Autodesk Inventor part; units mm, degrees
ref_plane "YZ Plane" through (0, 0, 0) normal (1, 0, 0) x (0, 1, 0)
ref_plane "XZ Plane" through (0, 0, 0) normal (0, 1, 0) x (-1, 0, 0)
ref_plane "XY Plane" through (0, 0, 0) normal (0, 0, 1) x (1, 0, 0)
sketch "Sketch1" plane through (0, 0, 0) normal (0, 0, 1) x (1, 0, 0)
  line L0 (0, 6.35) -> (0, 53.34)
  line L1 (0, 53.34) -> (-19.05, 53.34)
  line L2 (-19.05, 53.34) -> (-19.05, 55.245)
  line L3 (-12.7, 48.895) -> (-6.35, 48.895)
  line L4 (-6.35, 48.895) -> (-6.35, 13.335)
  line L5 (-6.35, 13.335) -> (-19.05, 13.335)
  line L6 (-19.05, 13.335) -> (-19.05, 12.7)
  line L7 (-12.7, 8.89) -> (-6.35, 8.89)
  line L8 (-6.35, 8.89) -> (-6.35, 0)
  line L9 (-6.35, 0) -> (0, 0)
  line L10 (-19.05, 55.245) -> (-19.05, 40.005)
  line L11 (-19.05, 40.005) -> (-12.7, 40.005)
  line L12 (-12.7, 40.005) -> (-12.7, 48.895)
  line L13 (-19.05, 12.7) -> (-19.05, 0)
  line L14 (-19.05, 0) -> (-12.7, 0)
  line L15 (-12.7, 0) -> (-12.7, 8.89)
  line L16 (0, 0) -> (0, 6.35)
  point P0 (-19.05, 53.34)
  point P1 (-19.05, 11.43)
  dimension "d1" = 35.56
  dimension "d2" = 4.445
  dimension "d3" = 4.445
  dimension "d4" = 6.35
  dimension "d6" = 6.35
  dimension "d7" = 6.35
  dimension "d13" = 13.335
  dimension "d14" = 13.335
extrude "Extrusion1" add sketch "Sketch1" along normal mid plane 3.81
sketch "Sketch4" plane through (0, 0, 0) normal (0, 0, 1) x (1, 0, 0)
  line L0 (0, 0) -> (-6.35, 0)
  line L1 (-6.35, 0) -> (25.4, 0)
  line L2 (25.4, 0) -> (25.4, 6.35)
  line L3 (25.4, 6.35) -> (-6.35, 6.35)
  line L4 (-6.35, 6.35) -> (-6.35, 0)
  dimension "d23" = 31.75
  dimension "d24" = 6.35
extrude "Extrusion4" add sketch "Sketch4" against normal mid plane 35.56
sketch "Sketch5" plane through (-6.35, 6.35, 17.78) normal (0, 1, 0) x (1, 0, 0)
  line L0 (31.75, 35.56) -> (0, 35.56) construction
  line L1 (6.35, 35.56) -> (6.35, 0) construction
  line L2 (31.75, 0) -> (0, 0) construction
  line L3 (31.75, 35.56) -> (31.75, 0) construction
  line L4 (6.35, 35.56) -> (31.75, 0) construction
  line L5 (31.75, 0) -> (6.35, 0) construction
  line L6 (31.75, 35.56) -> (6.35, 0) construction
  circle A0 centre (19.05, 17.78) radius 6.35
  point P0 (6.35, 17.78)
  dimension "d27" = 12.7
extrude "Extrusion5" cut sketch "Sketch5" against normal through all
fillet "Fillet2" radius 3.175 4 edges at (-6.35, 3.175, 17.78) (25.4, 3.175, 17.78) (25.4, 3.175, -17.78) (-6.35, 3.175, -17.78)
equation "\"d11\" = width"
equation "\"width\" = 3.81"
properties part number "round_0_5_inchHoleV01"
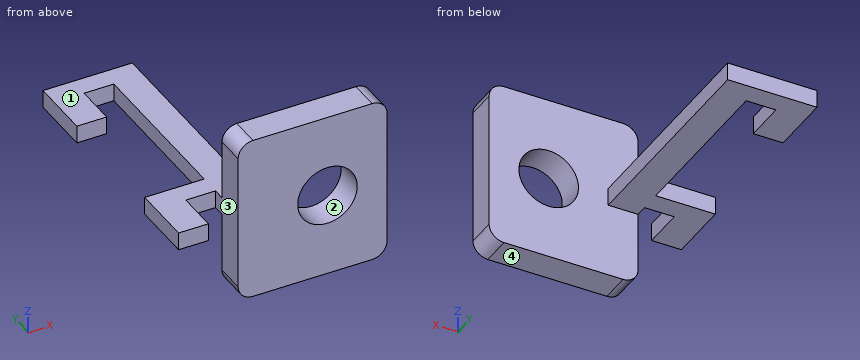
Verification items for the finished model (mm, model axes). Face numbers are marked on the shaded views. Coordinates: 2 decimals unless noted, no trailing zeros. Write each loop counter-clockwise with the first axis right and the second up, starting at its lowest first coordinate (ties: lowest second). Pieces come first, ordered by that corner, then holes. Notation, with made-up numbers: M -38,71 L -10,71 A21 ccw -10,103 Z; hole C -0.75,49.5 d8. An arc over 180 degrees is marked long. Use a Markdown table: item, result.
Q1. Sectioned sample at A-A, the plane z = 0. Record the boundary of the cut face in (x, y) (3 decimals).
Reply:
| item | result |
|---|---|
| outline | M -19.05,0 L -12.7,0 L -12.7,8.89 L -6.35,8.89 L -6.35,0 L 6.35,0 L 6.35,6.35 L 0,6.35 L 0,53.34 L -19.05,53.34 L -19.05,40.005 L -12.7,40.005 L -12.7,48.895 L -6.35,48.895 L -6.35,13.335 L -19.05,13.335 Z; M 19.05,0 L 25.4,0 L 25.4,6.35 L 19.05,6.35 Z |
Q2. Sectioned sample at C-C, the plane y = 43. Record the boundary of the cut face in (x, z) (3 decimals).
Reply:
| item | result |
|---|---|
| outline | M -19.05,-1.905 L -12.7,-1.905 L -12.7,1.905 L -19.05,1.905 Z; M -6.35,-1.905 L 0,-1.905 L 0,1.905 L -6.35,1.905 Z |
Q3. Thickness scan on line 1 (X direction, y = 4.5, z = 0); line 2 (Y direction, x = 20, z = -2); line 3 (Z direction, x = 12.7, y = 2.5). Record the ranges inside material, lowest first.
Reply:
| item | result |
|---|---|
| line 1 | x = -19.05 to -12.7, -6.35 to 6.35, 19.05 to 25.4 |
| line 2 | y = 0 to 6.35 |
| line 3 | z = -17.78 to -6.35, 6.35 to 17.78 |
Q4. Sectioned sample at D-D, the plane y = 31. Record the boundary of the cut face in (x, z) (3 decimals).
Reply:
| item | result |
|---|---|
| outline | M -6.35,-1.905 L 0,-1.905 L 0,1.905 L -6.35,1.905 Z |
Q5. Sectioned sample at B-B, the plane x = -7.5. Record the boundary of the cut face in (y, z) (3 decimals).
Reply:
| item | result |
|---|---|
| outline | M 8.89,-1.905 L 13.335,-1.905 L 13.335,1.905 L 8.89,1.905 Z; M 48.895,-1.905 L 53.34,-1.905 L 53.34,1.905 L 48.895,1.905 Z |
Q6. Draft check along Z on the marked faces 1, 2, 3 and 4. Enter one of: +Z half, -Z half, draft (parallel to the pull), parting line (faces both ways), or undercut.
Reply:
| item | result |
|---|---|
| face 1 | +Z half |
| face 2 | undercut |
| face 3 | draft |
| face 4 | -Z half |
Q7. Go/stop test with flat-tipped pins: P1, Ø4, axis at x = -10, z = -1, coming from the -Y side; P2, Ø4, axis at x = -1, z = 12.5, coming from the +Y side; P3, Ø15, axis at x = -9.5, y = 26, coming from the -Z side (3 decimals); P4, Ø9.5, axis at x = 13, z = 1.5, coming from the +Y side. Record where each tip stops, or that it passes through.
Reply:
| item | result |
|---|---|
| P1 | stops at y = 8.89 |
| P2 | stops at y = 6.35 |
| P3 | stops at z = -1.905 |
| P4 | passes through |
